```python
from build123d import *

# Parameters (mm, degrees)
SKETCH1_W           = 203.2
SKETCH1_H           = 127
BOSS_EXTRUDE1_DEPTH = 25.4
SKETCH2_W           = 199.644
SKETCH2_H           = 123.444
CUT_EXTRUDE1_DEPTH  = 22.86
SKETCH4_W           = 11.176
SKETCH4_H           = 12.192
SKETCH4_H_2         = 9.144
CUT_EXTRUDE2_DEPTH  = 1.778


with BuildPart() as part:
    # Sketch1 → Boss-Extrude1 (new body)
    with BuildSketch(Plane.XY):
        with Locations((101.6, 63.5)):
            Rectangle(SKETCH1_W, SKETCH1_H)
    extrude(amount=BOSS_EXTRUDE1_DEPTH)

    # Sketch2 → Cut-Extrude1 (cut)
    with BuildSketch(Plane.XY.offset(25.4)):
        with Locations((101.6, 63.5)):
            Rectangle(SKETCH2_W, SKETCH2_H)
    extrude(amount=-CUT_EXTRUDE1_DEPTH, mode=Mode.SUBTRACT)

    # Sketch4 → Cut-Extrude2 (cut)
    with BuildSketch(Plane.ZY):
        with Locations((10.414, 87.206902012)):
            Rectangle(SKETCH4_W, SKETCH4_H)
        with Locations((10.414, 36.152902012)):
            Rectangle(SKETCH4_W, SKETCH4_H_2)
    extrude(amount=-CUT_EXTRUDE2_DEPTH, mode=Mode.SUBTRACT)


solid = part.part
```
Geometry: final body of the model. Coordinates: model frame, mm. A direction names the side the tool comes from. Round coordinates to 2 decimals unless told otherwise and drop trailing zeros. Order: outer loops, then holes, each group sorted by start corner. A loop starts at its lowest first (then second) coordinate and runs counter-clockwise, first axis right, second up. Notation, with made-up numbers: M 76.25,74.5 L 106.25,74.5 A19 cw 106.25,82.5 Z; hole C 34,16 d3. An arc over 180 degrees is marked long. One line per item, written item: value.
(1) Reachability of faces 5 (the flat face through (100, 0, 13)), 6 (the flat face through (201.422, 63, 14)) from +Z, -Z, +X, -X, +Y, -Y: full face, straight path, thin tool, end or side. Return the list, or none.
Result sheet:
face 5: +Z, -Z, +X, -X, -Y
face 6: +Z
(2) Cut plane A-A (z = 13.5). Return the cut outline in (x, y).
Result sheet:
outline: M 0,0 L 203.2,0 L 203.2,127 L 0,127 L 0,93.3 L 1.78,93.3 L 1.78,125.22 L 201.42,125.22 L 201.42,1.78 L 1.78,1.78 L 1.78,31.58 L 0,31.58 Z; M 0,40.72 L 1.78,40.72 L 1.78,81.11 L 0,81.11 Z
(3) Cut plane B-B (y = 89). Return the cut outline in (x, z), and give its area (3 significant figures).
Result sheet:
outline: M 0,0 L 203.2,0 L 203.2,25.4 L 201.42,25.4 L 201.42,2.54 L 1.78,2.54 L 1.78,4.83 L 0,4.83 Z; M 0,16 L 1.78,16 L 1.78,25.4 L 0,25.4 Z
area: 578 mm2
(4) Cut plane C-C (z = 23.25). Return the cut outline in (x, y), and give its area (3 significant figures).
Result sheet:
outline: M 0,0 L 203.2,0 L 203.2,127 L 0,127 Z; hole M 1.78,1.78 L 201.42,1.78 L 201.42,125.22 L 1.78,125.22 Z
area: 1,160 mm2
(5) Line query: probe 1 along X at (y, z) = (97, 14); probe 2 along Y at (x, z) = (11.5, 13.5); probe 3 along Z at (x, y) = (191.5, 102). Output: solid intervals per line, ascending. Write a range as [from, to].
Result sheet:
probe 1: [0, 1.78], [201.42, 203.2]
probe 2: [0, 1.78], [125.22, 127]
probe 3: [0, 2.54]
(6) Pin query (flat end, axial travel): P1, Ø2, axis at x = 80, y = 23.5, coming from the +Z side. Return the tip coordinate at first contact, or that it passes through.
Result sheet:
P1: z = 2.54
(7) Pull-direction query (Y, two-part tool) for faces 1 (the flat face through (100, 127, 13)), 2 (the flat face through (100, 125.222, 14)), 3 (the flat face through (1.778, 63, 14)), 4 (the flat face through (203.2, 63, 13)); classes: pulls with the +Y half, pulls with the -Y half, needs draft (parallel to the pull), parting line crosses it, or undercut.
Result sheet:
face 1: pulls with the +Y half
face 2: undercut
face 3: undercut
face 4: needs draft
(8) Cut plane D-D (x = 117.5). Return the cut outline in (y, z).
Result sheet:
outline: M 0,0 L 127,0 L 127,25.4 L 125.22,25.4 L 125.22,2.54 L 1.78,2.54 L 1.78,25.4 L 0,25.4 Z
